```python
from build123d import *

# Parameters (mm, degrees)
BOSS_EXTRUDE1_DEPTH                                 = 10
CSK_FOR_M4_COUNTERSUNK_FLAT_HEAD_SCREW1_D           = 4.4
CSK_FOR_M4_COUNTERSUNK_FLAT_HEAD_SCREW1_DEPTH       = 10
CSK_FOR_M4_COUNTERSUNK_FLAT_HEAD_SCREW1_CSINK_D     = 9.4
CSK_FOR_M4_COUNTERSUNK_FLAT_HEAD_SCREW1_CSINK_ANGLE = 90
CSK_FOR_M4_COUNTERSUNK_FLAT_HEAD_SCREW1_TIP         = 1.321893362
SKETCH4_W                                           = 33
SKETCH4_H                                           = 22.7
SKETCH4_W_2                                         = 22.8
SKETCH4_H_2                                         = 12.5
EXTRUDE_THIN1_DEPTH                                 = 17.5
FILLET1_R                                           = 5
F_1_5MM_DOWEL_HOLE1_D                               = 1.8
F_1_5MM_DOWEL_HOLE1_DEPTH                           = 10
F_1_5MM_DOWEL_HOLE1_TIP                             = 0.540774557
SKETCH8_W                                           = 3
SKETCH8_H                                           = 12.5
CUT_EXTRUDE1_DEPTH                                  = 100.184172124
BOSS_EXTRUDE3_DEPTH                                 = 10
FILLET2_R                                           = 2


with BuildPart() as part:
    # Sketch1 → Boss-Extrude1 (new body)
    with BuildSketch(Plane(origin=(0, 0, 0), x_dir=(0, 1, 0), z_dir=(0, 0, 1))):
        with BuildLine():
            Line((-60, 62.5), (60, 62.5))
            ThreePointArc((60, 62.5), (70.606601718, 58.106601718), (75, 47.5))
            Line((75, 47.5), (75, -47.5))
            ThreePointArc((75, -47.5), (70.606601718, -58.106601718), (60, -62.5))
            Line((60, -62.5), (-60, -62.5))
            ThreePointArc((-60, -62.5), (-70.606601718, -58.106601718), (-75, -47.5))
            Line((-75, -47.5), (-75, 47.5))
            ThreePointArc((-75, 47.5), (-70.606601718, 58.106601718), (-60, 62.5))
        make_face()
    extrude(amount=BOSS_EXTRUDE1_DEPTH)

    # CSK for M4 Countersunk Flat Head Screw1
    with Locations(Plane(origin=(0, 0, 10), x_dir=(0, -1, 0), z_dir=(0, 0, 1))):
        with Locations((-67.11, 54.61), (67.11, 54.61), (67.11, -54.61), (-67.11, -54.61)):
            CounterSinkHole(CSK_FOR_M4_COUNTERSUNK_FLAT_HEAD_SCREW1_D / 2, CSK_FOR_M4_COUNTERSUNK_FLAT_HEAD_SCREW1_CSINK_D / 2, depth=CSK_FOR_M4_COUNTERSUNK_FLAT_HEAD_SCREW1_DEPTH, counter_sink_angle=CSK_FOR_M4_COUNTERSUNK_FLAT_HEAD_SCREW1_CSINK_ANGLE)
            with Locations((0, 0, -(CSK_FOR_M4_COUNTERSUNK_FLAT_HEAD_SCREW1_DEPTH + CSK_FOR_M4_COUNTERSUNK_FLAT_HEAD_SCREW1_TIP / 2))):  # 118° drill point
                Cone(0, CSK_FOR_M4_COUNTERSUNK_FLAT_HEAD_SCREW1_D / 2, CSK_FOR_M4_COUNTERSUNK_FLAT_HEAD_SCREW1_TIP, mode=Mode.SUBTRACT)

    # Sketch4 → Extrude-Thin1 (add)
    with BuildSketch(Plane.XY.offset(10)):
        Rectangle(SKETCH4_W, SKETCH4_H)
        Rectangle(SKETCH4_W_2, SKETCH4_H_2, mode=Mode.SUBTRACT)
    extrude(amount=EXTRUDE_THIN1_DEPTH)

    # Fillet1
    fillet1_edges = [part.edges().sort_by_distance(p)[0] for p in [
        (16.5, -11.35, 18.75),
        (16.5, 11.35, 18.75),
        (-16.5, 11.35, 18.75),
        (-16.5, -11.35, 18.75),
    ]]
    fillet(fillet1_edges, radius=FILLET1_R)

    # Ø1.5mm Dowel Hole1
    with Locations(Plane(origin=(0, 0, 27.5), x_dir=(0, -1, 0), z_dir=(0, 0, 1))):
        with Locations((0, -13.75), (0, 13.75)):
            Hole(F_1_5MM_DOWEL_HOLE1_D / 2, depth=F_1_5MM_DOWEL_HOLE1_DEPTH)
            with Locations((0, 0, -(F_1_5MM_DOWEL_HOLE1_DEPTH + F_1_5MM_DOWEL_HOLE1_TIP / 2))):  # 118° drill point
                Cone(0, F_1_5MM_DOWEL_HOLE1_D / 2, F_1_5MM_DOWEL_HOLE1_TIP, mode=Mode.SUBTRACT)

    # Sketch8 → Cut-Extrude1 (cut, through all)
    with BuildSketch(Plane.XY.offset(10)):
        with BuildLine():
            Line((-47.370334328, 43.972462246), (-47.370334328, -43.972462246))
            ThreePointArc((-47.370334328, -43.972462246), (-41.973713961, -49.369082612), (-36.577093595, -43.972462245))
            Line((-36.577093595, -43.972462245), (-36.577093595, 43.972462246))
            ThreePointArc((-36.577093595, 43.972462246), (-41.973713962, 49.369082612), (-47.370334328, 43.972462246))
        make_face()
        with BuildLine():
            Line((36.577093595, 43.972462246), (36.577093595, -43.972462245))
            ThreePointArc((36.577093595, -43.972462245), (41.973713961, -49.369082612), (47.370334328, -43.972462246))
            Line((47.370334328, -43.972462246), (47.370334328, 43.972462246))
            ThreePointArc((47.370334328, 43.972462246), (41.973713962, 49.369082612), (36.577093595, 43.972462246))
        make_face()
        Polygon((20, 61.232201212), (15.268419991, 57.794507111), (17.075722734, 52.232201212), (22.924277266, 52.232201212), (24.731580009, 57.794507111), align=None)
        Polygon((0, 61.232201212), (-4.731580009, 57.794507111), (-2.924277266, 52.232201212), (2.924277266, 52.232201212), (4.731580009, 57.794507111), align=None)
        with Locations((-9.9, 0)):
            Rectangle(SKETCH8_W, SKETCH8_H)
        Polygon((20, 45.791100606), (15.268419991, 42.353406505), (17.075722734, 36.791100606), (22.924277266, 36.791100606), (24.731580009, 42.353406505), align=None)
        Polygon((20, 30.35), (15.268419991, 26.912305899), (17.075722734, 21.35), (22.924277266, 21.35), (24.731580009, 26.912305899), align=None)
        Polygon((0, 45.791100606), (-4.731580009, 42.353406505), (-2.924277266, 36.791100606), (2.924277266, 36.791100606), (4.731580009, 42.353406505), align=None)
        Polygon((0, 30.35), (-4.731580009, 26.912305899), (-2.924277266, 21.35), (2.924277266, 21.35), (4.731580009, 26.912305899), align=None)
        Polygon((-24.731580009, 26.912305899), (-20, 30.35), (-15.268419991, 26.912305899), (-17.075722734, 21.35), (-22.924277266, 21.35), align=None)
        Polygon((-24.731580009, 42.353406505), (-20, 45.791100606), (-15.268419991, 42.353406505), (-17.075722734, 36.791100606), (-22.924277266, 36.791100606), align=None)
        Polygon((-24.731580009, 57.794507111), (-20, 61.232201212), (-15.268419991, 57.794507111), (-17.075722734, 52.232201212), (-22.924277266, 52.232201212), align=None)
        Polygon((24.731580009, -26.912305899), (20, -30.35), (15.268419991, -26.912305899), (17.075722734, -21.35), (22.924277266, -21.35), align=None)
        Polygon((4.731580009, -26.912305899), (0, -30.35), (-4.731580009, -26.912305899), (-2.924277266, -21.35), (2.924277266, -21.35), align=None)
        Polygon((-22.924277266, -21.35), (-24.731580009, -26.912305899), (-20, -30.35), (-15.268419991, -26.912305899), (-17.075722734, -21.35), align=None)
        Polygon((-22.924277266, -36.791100606), (-24.731580009, -42.353406505), (-20, -45.791100606), (-15.268419991, -42.353406505), (-17.075722734, -36.791100606), align=None)
        Polygon((4.731580009, -42.353406505), (0, -45.791100606), (-4.731580009, -42.353406505), (-2.924277266, -36.791100606), (2.924277266, -36.791100606), align=None)
        Polygon((24.731580009, -42.353406505), (20, -45.791100606), (15.268419991, -42.353406505), (17.075722734, -36.791100606), (22.924277266, -36.791100606), align=None)
        Polygon((24.731580009, -57.794507111), (20, -61.232201212), (15.268419991, -57.794507111), (17.075722734, -52.232201212), (22.924277266, -52.232201212), align=None)
        Polygon((4.731580009, -57.794507111), (0, -61.232201212), (-4.731580009, -57.794507111), (-2.924277266, -52.232201212), (2.924277266, -52.232201212), align=None)
        Polygon((-22.924277266, -52.232201212), (-24.731580009, -57.794507111), (-20, -61.232201212), (-15.268419991, -57.794507111), (-17.075722734, -52.232201212), align=None)
    extrude(amount=-CUT_EXTRUDE1_DEPTH, mode=Mode.SUBTRACT)

    # Sketch9 → Boss-Extrude3 (add)
    with BuildSketch(Plane(origin=(0, 0, 0), x_dir=(1, 0, 0), z_dir=(0, 0, -1))):
        with BuildLine():
            Line((-52.5, 80), (52.5, 80))
            ThreePointArc((52.5, 80), (63.106601718, 75.606601718), (67.5, 65))
            Line((67.5, 65), (67.5, -65))
            ThreePointArc((67.5, -65), (63.106601718, -75.606601718), (52.5, -80))
            Line((52.5, -80), (-52.5, -80))
            ThreePointArc((-52.5, -80), (-63.106601718, -75.606601718), (-67.5, -65))
            Line((-67.5, -65), (-67.5, 65))
            ThreePointArc((-67.5, 65), (-63.106601718, 75.606601718), (-52.5, 80))
        make_face()
        with BuildLine():
            Line((-47.5, 75), (47.5, 75))
            ThreePointArc((47.5, 75), (58.106601718, 70.606601718), (62.5, 60))
            Line((62.5, 60), (62.5, -60))
            ThreePointArc((62.5, -60), (58.106601718, -70.606601718), (47.5, -75))
            Line((47.5, -75), (-47.5, -75))
            ThreePointArc((-47.5, -75), (-58.106601718, -70.606601718), (-62.5, -60))
            Line((-62.5, -60), (-62.5, 60))
            ThreePointArc((-62.5, 60), (-58.106601718, 70.606601718), (-47.5, 75))
        make_face(mode=Mode.SUBTRACT)
    extrude(amount=-BOSS_EXTRUDE3_DEPTH)

    # Fillet2
    fillet2_edges = [part.edges().sort_by_distance(p)[0] for p in [
        (63.106601718, 75.606601718, 10),
        (0, 80, 10),
        (-63.106601718, 75.606601718, 10),
        (-67.5, 0, 10),
        (-63.106601718, -75.606601718, 10),
        (0, -80, 10),
        (63.106601718, -75.606601718, 10),
        (67.5, 0, 10),
    ]]
    fillet(fillet2_edges, radius=FILLET2_R)


solid = part.part
```
Build history of the part. All positions in model axes, mm. A direction names the side the tool comes from. Round coordinates to 2 decimals unless told otherwise and drop trailing zeros. Loops run counter-clockwise (first coordinate to the right, second up) from the corner with the lowest first, then second, coordinate; pieces in that order, holes last.
Item 1: Saw through at B-B (y = -23.5). List the corners of the cut face in (x, z).
Item 2: Saw through at A-A (z = 15). List the corners of the cut face in (x, y), then the cut area to 3 significant figures.
Item 3: Saw through at C-C (x = -54.61). State how many separate pieces and enclosed holes the cut face has, then the cut area to 3 significant figures.
Item 4: Two-plate mould, pull along X, no slides. Class faces 3 (the face through (-15.07, 9.85, 18.87)), 4 (the face through (-16.16, 24.17, 5.07)), 5 (the face through (1, -18, 10)): released by +X, released by -X, zero draft, split by the parting line, or undercut.
Item 5: Drill centre lines: line 1 along X through (y, z) = (10.5, 8.25); line 2 along Y through (x, z) = (5.5, 19); line 3 along Y through (x, z) = (54.61, 4.75). Where is each one in solid material? Low to high.
Item 6: Which spindle directions (+Z, -Z, +X, -X, +Y, -Y) get a long thin tool onto all of the face, cutting with end or side? Do faces 1 (the face through (0, 36.791, 5)), 2 (the face through (67.5, -1, 4)). Say none if no direction does.
Item 7: Pin check, flat tips, straight feed: P1, Ø5, axis at x = 29, y = 29, coming from the +Z side; P2, Ø5, axis at x = -54.61, y = -67.11, coming from the +Z side; P3, Ø12, axis at y = 43.5, z = 15, coming from the +X side; P4, Ø3.5, axis at x = -54.61, y = 67.11, coming from the -Z side. Stop position of each tip, or through.
Worked answers:
1. outline: (-67.5, 0) - (-47.37, 0) - (-47.37, 10) - (-65.5, 10) arc R2 ccw to (-67.5, 8) - close; (-36.58, 0) - (-23.62, 0) - (-23.62, 10) - (-36.58, 10) - close; (-16.38, 0) - (-3.62, 0) - (-3.62, 10) - (-16.38, 10) - close; (3.62, 0) - (16.38, 0) - (16.38, 10) - (3.62, 10) - close; (23.62, 0) - (36.58, 0) - (36.58, 10) - (23.62, 10) - close; (47.37, 0) - (67.5, 0) - (67.5, 8) arc R2 ccw to (65.5, 10) - (47.37, 10) - close
2. outline: (-16.5, -6.35) arc R5 ccw to (-11.5, -11.35) - (11.5, -11.35) arc R5 ccw to (16.5, -6.35) - (16.5, 6.35) arc R5 ccw to (11.5, 11.35) - (-11.5, 11.35) arc R5 ccw to (-16.5, 6.35) - close; hole (-11.4, -6.25) - (11.4, -6.25) - (11.4, 6.25) - (-11.4, 6.25) - close
2. area: 443 mm2
3. separate pieces: 3
3. enclosed holes: 0
3. area: 1,490 mm2
4. face 3: released by -X
4. face 4: undercut
4. face 5: zero draft
5. line 1: x = -67.48 to -47.37, -36.58 to 36.58, 47.37 to 67.48
5. line 2: y = -11.35 to -6.25, 6.25 to 11.35
5. line 3: y = -79.85 to -69.31, -64.91 to 64.91, 69.31 to 79.85
6. face 1: +Z, -Z
6. face 2: +Z, -Z, +X, +Y, -Y
7. P1: stops at z = 10
7. P2: stops at z = 7.8
7. P3: stops at x = 67.23
7. P4: passes through
